Geometry: final body of the model. Coordinates: model frame, mm. A direction names the side the tool comes from. Coordinates: 2 decimals unless noted, no trailing zeros. Write each loop counter-clockwise with the first axis right and the second up, starting at its lowest first coordinate (ties: lowest second). Pieces come first, ordered by that corner, then holes. Notation, with made-up numbers: M -16.75,-39 L -6.75,-39 A22 cw -6.75,-5 Z; hole C 19,-3 d10. An arc over 180 degrees is marked long. Write item = value, one per line. Start each with the question number.
Item 1: Ray query, L1, parallel to X at y = -57.5, z = 3.5; L2, parallel to Y at x = 78.5, z = 2.5; L3, parallel to Y at x = -13.5, z = 2.25. Return the intervals inside material, ascending. Write a range as [from, to].
Item 2: Section C-C on z = 4.25. Give the number of separate pieces and of enclosed holes in the cut face, plus the area to 3 significant figures.
Item 3: Section B-B on x = 23. Output: boundary loops of the cut face in (y, z).
Item 4: Reachability of faces 4 (the flat face through (85, 57, 7)), 5 (the flat face through (85, -56, 7)), 6 (the flat face through (-1, 52.5, 5)) from +Z, -Z, +X, -X, +Y, -Y: full face, straight path, thin tool, end or side. Return the list, or none.
Item 5: Section A-A on y = 7.5. Output: boundary loops of the cut face in (x, z), plus the area to 3 significant figures.
Item 6: Pull-direction query (X, two-part tool) for faces 1 (the flat face through (-82.5, -1, 5)), 2 (the flat face through (92, -1, 4)), 3 (the flat face through (-87, 1, 9)); classes: +X half, -X half, draft (parallel to the pull), parting line (faces both ways), or undercut.
Item 7: First-contact query: pin 1 Ø2 at (y, z) = (-60, 8.5) entering from +X; pin 2 Ø20 at (x, y) = (85, 58.5) entering from +Z; pin 3 Ø3 at (x, y) = (78.5, -57.5) entering from +Z; pin 4 Ø1 at (x, z) = (-89.5, 8) entering from +Y. Flat tips, straight axial feed; report the tip coordinate or a pass-through.
from build123d import *

# Parameters (mm, degrees)
F0_W        = 184
F0_H        = 128
F1_DEPTH    = 7
F2_W        = 165
F2_H        = 105
F3_DEPTH    = 7
F4_W        = 74
F4_H        = 11.5
F5_DEPTH    = 2
F6_T1_DEPTH = 32.4
F7_W        = 9.5
F7_H        = 44.45
F8_DEPTH    = 2
F10_DEPTH   = 7
F12_DEPTH   = 7


# Not quite as in the source:
# - a fillet or chamfer that OpenCascade refuses, or shapes differently, is made with other operations: its cross-section is extruded or revolved along the edge and cut away or added
# - a pattern or mirror of a feature is missing from the dataset's text; its kind, count and spacing are read off the source's solid


with BuildPart() as f1:
    # F0 (on Top) → F1 (new body)
    with BuildSketch(Plane.XY):
        Rectangle(F0_W, F0_H)
    extrude(amount=F1_DEPTH)

    # F2 (on face) → F3 (cut, through all)
    with BuildSketch(Plane.XY.offset(7)):
        Rectangle(F2_W, F2_H)
    extrude(amount=-F3_DEPTH, mode=Mode.SUBTRACT)

    # F4 (on face) → F5 (join)
    with BuildSketch(Plane.XY.offset(7)):
        with Locations((-37, 58.25)):
            Rectangle(F4_W, F4_H)
        with Locations((37, 58.25)):
            Rectangle(F4_W, F4_H)
        with Locations((-37, -58.25)):
            Rectangle(F4_W, F4_H)
        with Locations((37, -58.25)):
            Rectangle(F4_W, F4_H)
    extrude(amount=F5_DEPTH)

    # F6: fillet of radius 5.08 on 4 edges, made by hand

    # F6_s2 → F6_t1 (cut)
    with BuildSketch(Plane.XY.offset(-12.7)):
        with BuildLine():
            add(Edge.make_bspline(
                [(92, -58.92), (92, -64), (86.92, -64)],
                knots=[0, 0, 0, 1, 1, 1], degree=2, weights=[1, 1, 1]))
            Line((86.92, -64), (92, -64))
            Line((92, -64), (92, -58.92))
        make_face()
        with BuildLine():
            add(Edge.make_bspline(
                [(92, 58.92), (92, 64), (86.92, 64)],
                knots=[0, 0, 0, 1, 1, 1], degree=2, weights=[1, 1, 1]))
            Line((86.92, 64), (92, 64))
            Line((92, 64), (92, 58.92))
        make_face()
        with BuildLine():
            add(Edge.make_bspline(
                [(-86.92, 64), (-92, 64), (-92, 58.92)],
                knots=[0, 0, 0, 1, 1, 1], degree=2, weights=[1, 1, 1]))
            Line((-92, 58.92), (-92, 64))
            Line((-92, 64), (-86.92, 64))
        make_face()
        with BuildLine():
            add(Edge.make_bspline(
                [(-86.92, -64), (-92, -64), (-92, -58.92)],
                knots=[0, 0, 0, 1, 1, 1], degree=2, weights=[1, 1, 1]))
            Line((-92, -58.92), (-92, -64))
            Line((-92, -64), (-86.92, -64))
        make_face()
    extrude(amount=F6_T1_DEPTH, mode=Mode.SUBTRACT)

    # F7 (on face) → F8 (join)
    with BuildSketch(Plane.XY.offset(7)):
        with Locations((87.25, -22.225)):
            Rectangle(F7_W, F7_H)
        with Locations((87.25, 22.225)):
            Rectangle(F7_W, F7_H)
    f8 = extrude(amount=F8_DEPTH)

    # F8_copies: F8 across plane
    add(f8.mirror(Plane(origin=(0, 0, 0), x_dir=(0, 0, -1), z_dir=(-1, 0, 0))))

    # F9 (on face) → F10 (cut, through all)
    with BuildSketch(Plane.XY.offset(7)):
        with BuildLine():
            ThreePointArc((80.25, 57.5), (77.2625631329, 58.7374368671), (78.5, 55.75))
            ThreePointArc((78.5, 55.75), (79.7374368671, 56.2625631329), (80.25, 57.5))
        make_face()
    f10 = extrude(amount=-F10_DEPTH, mode=Mode.SUBTRACT)

    # F10_copies: F10 across plane
    add(f10.mirror(Plane(origin=(0, 0, 0), x_dir=(0, 0, -1), z_dir=(-1, 0, 0))), mode=Mode.SUBTRACT)

    # F11 (on face) → F12 (cut, through all)
    with BuildSketch(Plane(origin=(0, 0, 0), x_dir=(1, 0, 0), z_dir=(0, 0, -1))):
        with BuildLine():
            ThreePointArc((-76.75, 57.5), (-79.7374368671, 58.7374368671), (-78.5, 55.75))
            ThreePointArc((-78.5, 55.75), (-77.2625631329, 56.2625631329), (-76.75, 57.5))
        make_face()
        with BuildLine():
            ThreePointArc((80.25, 57.5), (77.2625631329, 58.7374368671), (78.5, 55.75))
            ThreePointArc((78.5, 55.75), (79.7374368671, 56.2625631329), (80.25, 57.5))
        make_face()
    extrude(amount=-F12_DEPTH, mode=Mode.SUBTRACT)


solid = f1.part
Responses:
q1.L1 = [-92, -80.25], [-76.75, 76.75], [80.25, 92]
q1.L2 = [-64, -59.25], [-55.75, -52.5], [52.5, 55.75], [59.25, 64]
q1.L3 = [-64, -52.5], [52.5, 64]
q2.separate_pieces = 1
q2.enclosed_holes = 5
q2.area = 6,170 mm²
q3.outline = M -64,0 L -52.5,0 L -52.5,9 L -64,9 Z; M 52.5,0 L 64,0 L 64,9 L 52.5,9 Z
q4.face_4 = +Z, +X, +Y
q4.face_5 = +Z, +X, -Y
q4.face_6 = +Z, -Z
q5.outline = M -92,0 L -82.5,0 L -82.5,9 L -92,9 Z; M 82.5,0 L 92,0 L 92,9 L 82.5,9 Z
q5.area = 171 mm²
q6.face_1 = undercut
q6.face_2 = +X half
q6.face_3 = draft
q7.pin_1 = 74
q7.pin_2 = 7
q7.pin_3 = through
q7.pin_4 = 44.45
